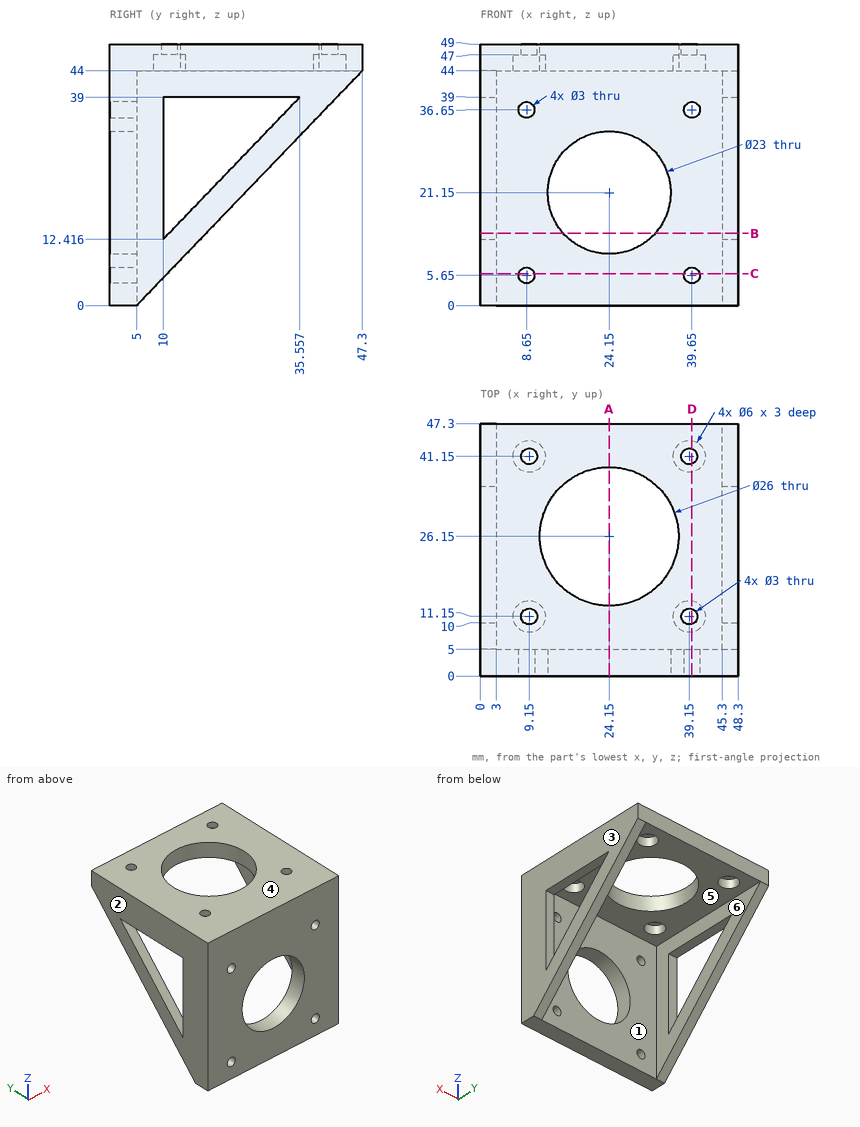
Geometry check sheet. Reference: drawing and pictorial views, mm from the part's lowest x, y, z. A direction names the side the tool comes from. Give positions to 0.01 mm unless a question says otherwise; leave off trailing zeros. Write each loop counter-clockwise with the first axis right and the second up, starting at its lowest first coordinate (ties: lowest second). Pieces come first, ordered by that corner, then holes. Notation, with made-up numbers: (-20, -25.5) -> (38, -25.5) arc R18 cw to (38, -7.5) -> close; hole circle Ø6 at (3, 21). An arc over 180 degrees is marked (long way). One line per question, with ' | ' between items.
Item 1: Sectioned sample at D-D, the plane x = 39.65. State how many separate pieces and enclosed holes the cut face has.
Determined:
separate pieces: 5 | enclosed holes: 0
Item 2: Sectioned sample at B-B, the plane z = 13.5. Record the boundary of the cut face in (x, y).
Determined:
outline: (0, 0) -> (15.56, 0) -> (15.56, 5) -> (3, 5) -> (3, 10) -> (0, 10) -> close; (0, 11.04) -> (3, 11.04) -> (3, 17.98) -> (0, 17.98) -> close; (32.74, 0) -> (48.3, 0) -> (48.3, 10) -> (45.3, 10) -> (45.3, 5) -> (32.74, 5) -> close; (45.3, 11.04) -> (48.3, 11.04) -> (48.3, 17.98) -> (45.3, 17.98) -> close
Item 3: Sectioned sample at C-C, the plane z = 6. Record the boundary of the cut face in (x, y), plus the area to 3 significant figures.
Determined:
outline: (0, 0) -> (7.19, 0) -> (7.19, 5) -> (3, 5) -> (3, 10.77) -> (0, 10.77) -> close; (10.11, 0) -> (38.19, 0) -> (38.19, 5) -> (10.11, 5) -> close; (41.11, 0) -> (48.3, 0) -> (48.3, 10.77) -> (45.3, 10.77) -> (45.3, 5) -> (41.11, 5) -> close | area: 247 mm^2
Item 4: Depth check by flat-ended pin: pin 1 (0.9 mm diameter, centred on x = 47.5, z = 23.5, fed in from +Y) (1 decimal); pin 2 (10 mm diameter, centred on x = 25.5, y = 13, fed in from -Z); pin 3 (3.5 mm diameter, centred on x = 39.15, y = 11.15, fed in from -Z); pin 4 (1.8 mm diameter, centred on x = 39.65, z = 36.65, fed in from +Y). Enter the tip coordinate at first touch or a pass-through.
Determined:
pin 1: y = 28 | pin 2: z = 44 | pin 3: z = 47 | pin 4: through
Item 5: Sectioned sample at A-A, the plane x = 24.15. Record the boundary of the cut face in (y, z).
Determined:
outline: (0, 0) -> (5, 0) -> (5, 9.65) -> (0, 9.65) -> close; (0, 32.65) -> (5, 32.65) -> (5, 44) -> (13.15, 44) -> (13.15, 49) -> (0, 49) -> close; (39.15, 44) -> (47.3, 44) -> (47.3, 49) -> (39.15, 49) -> close
Item 6: Access from +Z, -Z, +X, -X, +Y, -Y to the whole of each face (thin tool, end or side, straight path). Record for the marked faces 1 and 2.
Determined:
face 1: -Z, +Y | face 2: +Z, -Z, -X, +Y, -Y
Item 7: Scan lines: line 1 along X through (y, z) = (2.85, 36.65); line 2 along X through (y, z) = (34, 43); line 3 along X through (y, z) = (11.15, 48.1). Record each from-to range of solid material in increasing order.
Determined:
line 1: 0 to 7.15, 10.15 to 38.15, 41.15 to 48.3 | line 2: 0 to 3, 45.3 to 48.3 | line 3: 0 to 7.65, 10.65 to 37.65, 40.65 to 48.3
Item 8: Draft check along X on the marked faces 3, 4, 5 and 6. Enter one of: released by +X, released by -X, zero draft, split by the parting line, or undercut.
Determined:
face 3: released by +X | face 4: zero draft | face 5: undercut | face 6: undercut
